Print and shaded views of the part. All mm, measured from the part's lowest x, y and z. A direction names the side the tool comes from. Give positions to 0.01 mm unless a question says otherwise; leave off trailing zeros. Order: outer loops, then holes, each group sorted by start corner. A loop starts at its lowest first (then second) coordinate and runs counter-clockwise, first axis right, second up. Notation, with made-up numbers: (-39.5, -15.5) -> (-9.5, -15.5) arc R19 cw to (-9.5, 8.5) -> close; hole circle Ø2 at (81, 17.5). An arc over 180 degrees is marked (long way). One line per question, with ' | ' between items. Start each with the question number.
(1) Cut at A-A (z = 17.3). Give the cut face in (x, y), then the cut area to 4 significant figures.
(2) Which spindle directions (+Z, -Z, +X, -X, +Y, -Y) get a long thin tool onto all of the face, cutting with end or side? Do the marked faces 4 and 5. Say none if no direction does.
(3) Cut at C-C (x = 17.3). Give the cut face in (y, z), then the cut area to 3 significant figures.
(4) Pin check, flat tips, straight feed: pin 1 Ø2.5 at (x, z) = (8.3, 17.3) entering from -Y; pin 2 Ø4 at (x, y) = (22, 2.5) entering from +Z; pin 3 Ø3 at (x, y) = (28.5, 7.5) entering from +Z. Stop position of each tip, or through.
(5) Cut at D-D (y = 3.75). Give the cut face in (x, z), then the cut area to 3 significant figures.
(6) Cut at B-B (x = 8.3). Give the cut face in (y, z), then the cut area to 3 significant figures.
(7) Drill centre lines: L1, parallel to X at y = 7.5, z = 17.3; L2, parallel to X at y = 2, z = 17.3; L3, parallel to Y at x = 30, z = 27.5. Where is each one in solid material? Low to high. Write a range as from..to.
(8) Pull direction Y, two halves, no side cores. Call the marked faces 1, 2 and 3: +Y half, -Y half, draft (parallel to the pull), parting line (faces both ways), or undercut.
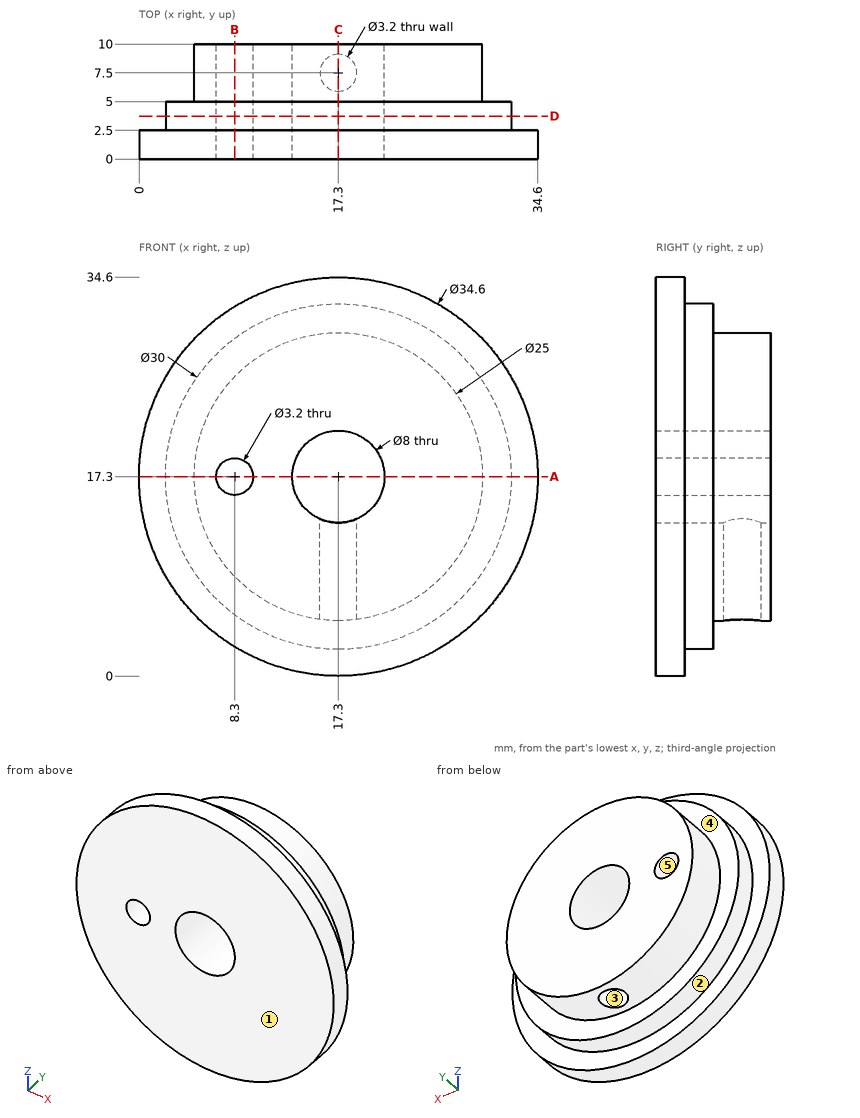
Result set:
1) outline: (0, 0) -> (6.7, 0) -> (6.7, 10) -> (4.8, 10) -> (4.8, 5) -> (2.3, 5) -> (2.3, 2.5) -> (0, 2.5) -> close; (9.9, 0) -> (13.3, 0) -> (13.3, 10) -> (9.9, 10) -> close; (21.3, 0) -> (34.6, 0) -> (34.6, 2.5) -> (32.3, 2.5) -> (32.3, 5) -> (29.8, 5) -> (29.8, 10) -> (21.3, 10) -> close | area: 174.5 mm2
2) face 4: +Y | face 5: +Y, -Y
3) outline: (0, 0) -> (2.5, 0) -> (2.5, 2.3) -> (5, 2.3) -> (5, 4.8) -> (5.9, 4.8) -> (5.9, 13.3) -> (0, 13.3) -> close; (0, 21.3) -> (10, 21.3) -> (10, 29.8) -> (5, 29.8) -> (5, 32.3) -> (2.5, 32.3) -> (2.5, 34.6) -> (0, 34.6) -> close; (9.1, 4.8) -> (10, 4.8) -> (10, 13.3) -> (9.1, 13.3) -> close | area: 179 mm2
4) pin 1: passes through | pin 2: stops at z = 34.39 | pin 3: stops at z = 25.18
5) outline: circle Ø30 at (17.3, 17.3); hole circle Ø3.2 at (8.3, 17.3); hole circle Ø8 at (17.3, 17.3) | area: 649 mm2
6) outline: (0, 2.53) -> (2.5, 2.53) -> (2.5, 5.3) -> (5, 5.3) -> (5, 8.63) -> (10, 8.63) -> (10, 15.7) -> (0, 15.7) -> close; (0, 18.9) -> (10, 18.9) -> (10, 25.97) -> (5, 25.97) -> (5, 29.3) -> (2.5, 29.3) -> (2.5, 32.07) -> (0, 32.07) -> close | area: 189 mm2
7) L1: x = 4.8..6.7, 9.9..13.3, 21.3..29.8 | L2: x = 0..6.7, 9.9..13.3, 21.3..34.6 | L3: y = 0..2.5
8) face 1: -Y half | face 2: draft | face 3: undercut
